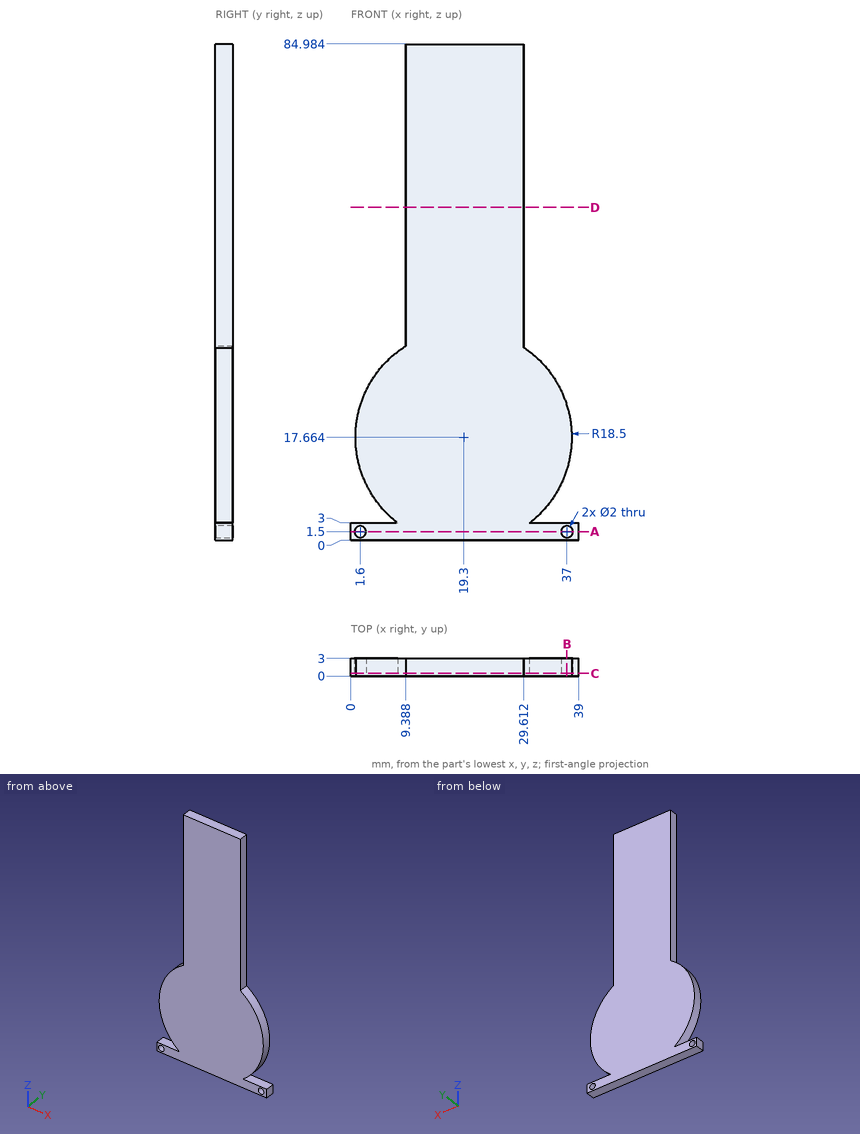
Here's the drawing with two shaded views (mm, measured from the low corner). I have some questions. Give positions to 0.01 mm unless a question says otherwise; leave off trailing zeros. Loops run counter-clockwise (first coordinate to the right, second up) from the corner with the lowest first, then second, coordinate; pieces in that order, holes last. Notation, with made-up numbers: M 62,36.25 L 101,36.25 A3 ccw 101,41.25 Z; hole C -4,74 d6. An arc over 180 degrees is marked long. Use one line per item in the form item = value. Start each with the question number.
(1) I want a section at C-C, the plane y = 0.45. Write out the boundary of the cut face in (x, z) (1 decimal).
(2) I want a section at D-D, the plane z = 57. Write out the boundary of the cut face in (x, y).
(3) I'm going to push flat-ended pins straight in: P1, Ø1.5, axis at y = 1, z = 68.5, coming from the +X side; P2, Ø1.6, axis at x = 37, z = 1.5, coming from the +Y side; P3, Ø1.5, axis at y = 2, z = 66.5, coming from the -X side. Where does each tip first touch, or does it pass through?
(4) I want a section at B-B, the plane x = 37. Write out the boundary of the cut face in (y, z) (1 decimal), and give its area (3 significant figures).
(5) I want a section at A-A, the plane z = 1.5. Write out the boundary of the cut face in (x, y).
(6) Please list where these lines run through material, in increasing order: line 1 (X direction, y = 2.25, z = 1.5); line 2 (Z direction, x = 2.5, y = 1.85) (1 decimal); line 3 (X direction, y = 2.1, z = 64.5).
Worked out:
q1.outline = M 0,0 L 39,0 L 39,3 L 30.6,3 A18.5 ccw 29.6,33 L 29.6,85 L 9.4,85 L 9.4,33.3 A18.5 ccw 8,3 L 0,3 Z; hole C 1.6,1.5 d2; hole C 37,1.5 d2
q2.outline = M 9.39,0 L 29.61,0 L 29.61,3 L 9.39,3 Z
q3.P1 = 29.61
q3.P2 = through
q3.P3 = 9.39
q4.outline = M 0,0 L 3,0 L 3,0.5 L 0,0.5 Z; M 0,2.5 L 3,2.5 L 3,3 L 0,3 Z; M 0,12.3 L 3,12.3 L 3,23 L 0,23 Z
q4.area = 35.3 mm²
q5.outline = M 0,0 L 0.6,0 L 0.6,3 L 0,3 Z; M 2.6,0 L 36,0 L 36,3 L 2.6,3 Z; M 38,0 L 39,0 L 39,3 L 38,3 Z
q6.line_1 = 0 to 0.6, 2.6 to 36, 38 to 39
q6.line_2 = 0 to 1.1, 1.9 to 3, 9.9 to 25.4
q6.line_3 = 9.39 to 29.61
